CAD build for the part. Positions are in the model's coordinates, mm. A direction names the side the tool comes from. Round coordinates to 2 decimals unless told otherwise and drop trailing zeros. Loops run counter-clockwise (first coordinate to the right, second up) from the corner with the lowest first, then second, coordinate; pieces in that order, holes last.
from build123d import *

# Parameters (mm, degrees)
F0_W     = 254
F0_H     = 76.2
F1_DEPTH = 6.35
F2_W     = 6.35
F2_H     = 6.35
F2_H_2   = 12.7
F2_H_3   = 31.75
F3_DEPTH = 6.35
F4_W     = 30.48
F4_H     = 6.35
F5_DEPTH = 6.351


with BuildPart() as f1:
    # F0 (on Front) → F1 (new body)
    with BuildSketch(Plane.XZ):
        with Locations((127, 38.1)):
            Rectangle(F0_W, F0_H)
    extrude(amount=F1_DEPTH)

    # F2 (on face) → F3 (cut, through all)
    with BuildSketch(Plane.XZ.offset(6.35)):
        with Locations((3.175, 3.175)):
            Rectangle(F2_W, F2_H)
        with Locations((3.175, 69.85)):
            Rectangle(F2_W, F2_H_2)
        with Locations((3.175, 34.925)):
            Rectangle(F2_W, F2_H_3)
        with Locations((250.825, 3.175)):
            Rectangle(F2_W, F2_H)
        with Locations((250.825, 34.925)):
            Rectangle(F2_W, F2_H_3)
        with Locations((250.825, 69.85)):
            Rectangle(F2_W, F2_H_2)
    extrude(amount=-F3_DEPTH, mode=Mode.SUBTRACT)

    # F4 (on face) → F5 (cut, through all)
    with BuildSketch(Plane.XZ.offset(6.35)):
        with Locations((15.24, 3.175)):
            Rectangle(F4_W, F4_H)
        with Locations((71.12, 3.175)):
            Rectangle(F4_W, F4_H)
        with Locations((127, 3.175)):
            Rectangle(F4_W, F4_H)
        with Locations((182.88, 3.175)):
            Rectangle(F4_W, F4_H)
        with Locations((238.76, 3.175)):
            Rectangle(F4_W, F4_H)
    extrude(amount=-F5_DEPTH, mode=Mode.SUBTRACT)


solid = f1.part
Item 1: Wall check: L1, parallel to X at y = -3.5, z = 73; L2, parallel to Z at x = 182, y = -3. Give the ranges that are in metal, low to high.
Verdict:
L1: x = 6.35 to 247.65
L2: z = 6.35 to 76.2
Item 2: Flat gauge pins, fed straight in: P1, Ø3, axis at y = -4.5, z = 2, coming from the -X side; P2, Ø1.5, axis at y = -3.5, z = 48.5, coming from the +X side; P3, Ø6, axis at x = 163.5, z = 8.5, coming from the +Y side; P4, Ø1.9, axis at y = -4, z = 72, coming from the -X side. Where does each tip first touch, or does it go through?
Verdict:
P1: stops at x = 30.48
P2: stops at x = 247.65
P3: stops at y = 0
P4: stops at x = 6.35
Item 3: Cut at C-C (x = 119). List the corners of the cut face in (y, z).
Verdict:
outline: (-6.35, 6.35) - (0, 6.35) - (0, 76.2) - (-6.35, 76.2) - close
Item 4: Mould opens along X. For faces 1 (the flat face through (125, -3, 76.2)), 2 (the flat face through (0, -3, 57)), 3 (the flat face through (254, -3, 13)), 4 (the flat face through (183, -3, 6.35)) say: released by +X, released by -X, zero draft, split by the parting line, or undercut.
Verdict:
face 1: zero draft
face 2: released by -X
face 3: released by +X
face 4: undercut
Item 5: Cut at B-B (z = 70). List the corners of the cut face in (x, y).
Verdict:
outline: (6.35, -6.35) - (247.65, -6.35) - (247.65, 0) - (6.35, 0) - close
Item 6: 3-axis set-ups, long thin cutter, end or side, ignore diameter. For faces 5 (the flat face through (251, -3, 63.5)), 6 (the flat face through (3, -3, 63.5)), 7 (the flat face through (71, -3, 6.35)): which of +Z, -Z, +X, -X, +Y, -Y reach the whole face in a straight line?
Verdict:
face 5: +Z, +X, +Y, -Y
face 6: +Z, -X, +Y, -Y
face 7: -Z, +Y, -Y
